Here's the drawing with two shaded views (mm, measured from the low corner). I have some questions. A direction names the side the tool comes from. Give positions to 0.01 mm unless a question says otherwise; leave off trailing zeros. Loops run counter-clockwise (first coordinate to the right, second up) from the corner with the lowest first, then second, coordinate; pieces in that order, holes last. Notation, with made-up numbers: (7, 43) -> (65, 43) arc R27 cw to (65, 80) -> close; hole circle Ø11 at (-8, 31). An arc over 180 degrees is marked (long way). Answer in a Markdown table with one row per item. Add a question column.
Item 1: If I drill on line 1 (X direction, y = 66.5, z = 1.5); line 2 (X direction, y = 59, z = 12); line 3 (Y direction, x = 57.5, z = 3.25) (1 decimal), over which ranges is the centre line in solid material (lowest first)?
Item 2: If we section it at A-A (y = 50): Write out the boundary of the cut face in (x, z), then the cut area to 3 significant figures.
Item 3: For P1, Ø3, axis at x = 89.5, z = 20, coming from the +Y side (1 decimal); P2, Ø10, axis at y = 51, z = 8, coming from the +X side; P3, Ø5, axis at y = 23.5, z = 12, coming from the +X side; P4, Ø8, axis at x = 45, z = 20.5, coming from the +Y side, each with a flat end and sliding along its axis, tell me the tip position at first contact or that it passes through.
Item 4: If we section it at C-C (z = 3.5): Write out the boundary of the cut face in (x, y).
Item 5: We'd pull the mould along X, two halves only. Please class the marked faces 1, 2 and 3: released by +X, released by -X, zero draft, split by the parting line, or undercut.
Item 6: If we section it at B-B (x = 50): Write out the boundary of the cut face in (y, z) (1 decimal).
Item 7: If we section it at D-D (z = 18.75): Write out the boundary of the cut face in (x, y).
Item 8: Which directions (+Z, -Z, +X, -X, +Y, -Y) give clear straight access to the entire face, cutting with the end or side of a thin tool? Please do the marked faces 4, 5 and 6.
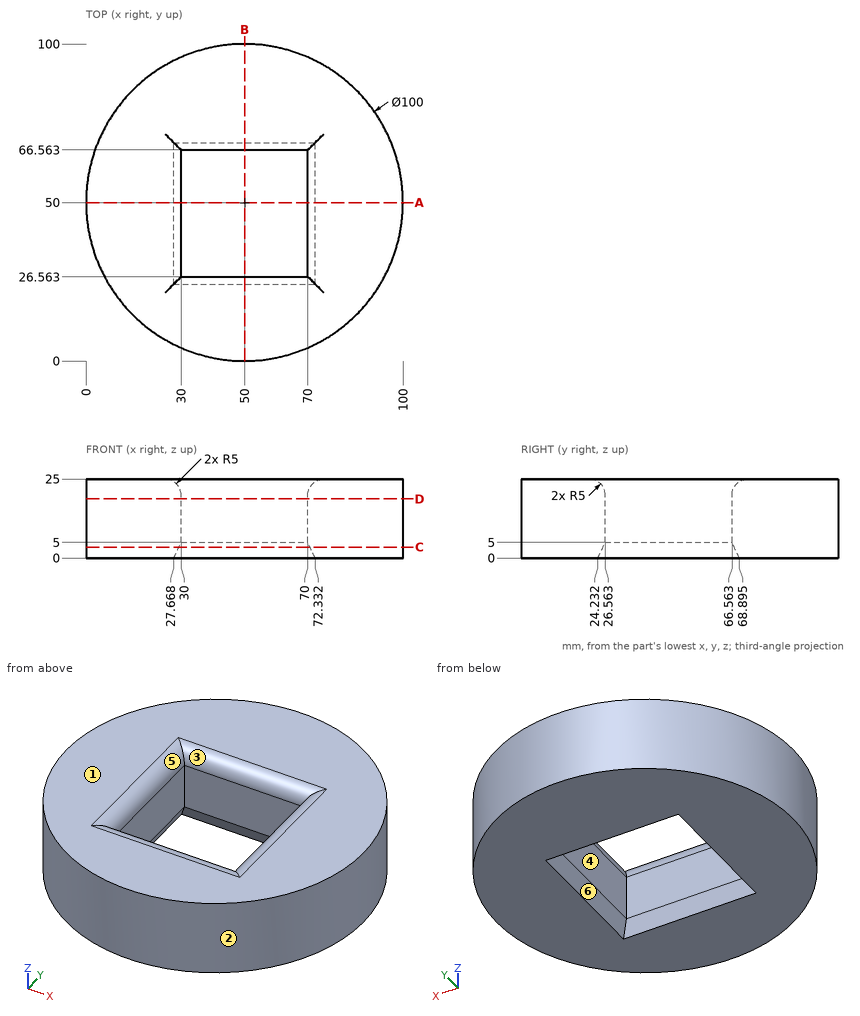
Recorded:
| question | item | result |
|---|---|---|
| 1 | line 1 | x = 2.8 to 28.37, 71.63 to 97.2 |
| 1 | line 2 | x = 0.82 to 30, 70 to 99.18 |
| 1 | line 3 | y = 0.6 to 25.7, 67.4 to 99.4 |
| 2 | outline | (0, 0) -> (27.67, 0) -> (30, 5) -> (30, 20) arc R5 ccw to (25, 25) -> (0, 25) -> close; (70, 5) -> (72.33, 0) -> (100, 0) -> (100, 25) -> (75, 25) arc R5 ccw to (70, 20) -> close |
| 2 | area | 1,480 mm^2 |
| 3 | P1 | stops at y = 82.5 |
| 3 | P2 | stops at x = 100 |
| 3 | P3 | stops at x = 93.86 |
| 3 | P4 | stops at y = 99.99 |
| 4 | outline | circle Ø100 at (50, 50); hole (29.3, 25.86) -> (70.7, 25.86) -> (70.7, 67.26) -> (29.3, 67.26) -> close |
| 5 | face 1 | zero draft |
| 5 | face 2 | split by the parting line |
| 5 | face 3 | undercut |
| 6 | outline | (0, 0) -> (24.2, 0) -> (26.6, 5) -> (26.6, 20) arc R5 ccw to (21.6, 25) -> (0, 25) -> close; (66.6, 5) -> (68.9, 0) -> (100, 0) -> (100, 25) -> (71.6, 25) arc R5 ccw to (66.6, 20) -> close |
| 7 | outline | circle Ø100 at (50, 50); hole (30, 26.56) -> (70, 26.56) -> (70, 66.56) -> (30, 66.56) -> close |
| 8 | face 4 | +Z, -Z |
| 8 | face 5 | +Z |
| 8 | face 6 | -Z |
